Here's the drawing with two shaded views (mm, measured from the low corner). I have some questions. Coordinates: 2 decimals unless noted, no trailing zeros. Write each loop counter-clockwise with the first axis right and the second up, starting at its lowest first coordinate (ties: lowest second). Pieces come first, ordered by that corner, then holes. Notation, with made-up numbers: (64.5, -32) -> (99.5, -32) arc R17 ccw to (99.5, -11) -> close; hole circle Ø5 at (74, -20). An arc over 180 degrees is marked (long way). Use one line per item in the form item = value.
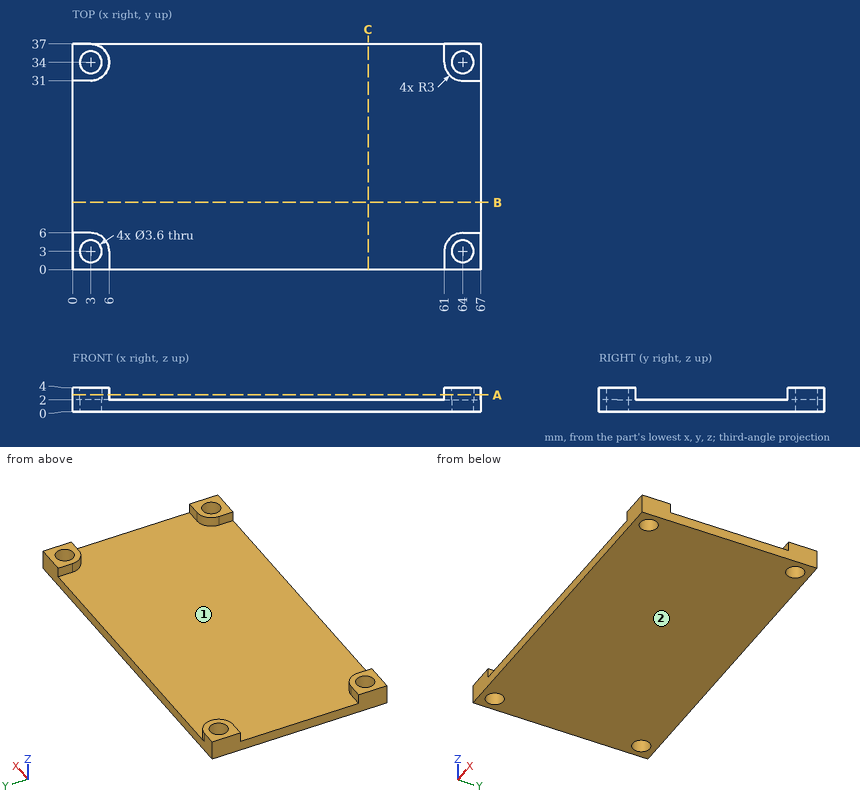
Q1. Suppose I cut it at B-B (y = 11). Write out the boundary of the cut face in (x, z), then the cut area to 3 significant figures.
Return value:
outline = (0, 0) -> (67, 0) -> (67, 2) -> (0, 2) -> close
area = 134 mm2
Q2. Suppose I cut it at C-C (x = 48.5). Write out the boundary of the cut face in (y, z).
Return value:
outline = (0, 0) -> (37, 0) -> (37, 2) -> (0, 2) -> close
Q3. If I drill on line 1 (Y direction, x = 64, z = 3.05); line 2 (Y direction, x = 3, z = 0.95); line 3 (X direction, y = 34, z = 1), over which ranges is the centre line in solid material (lowest first)? Write a range as from..to.
Return value:
line_1 = 0..1.2, 4.8..6, 31..32.2, 35.8..37
line_2 = 0..1.2, 4.8..32.2, 35.8..37
line_3 = 0..1.2, 4.8..62.2, 65.8..67
Q4. Thinking about a two-plate mould opening in X: for the marked faces 1 and 2, which applies, released by +X, released by -X, zero draft, split by the parting line, or undercut?
Return value:
face_1 = undercut
face_2 = zero draft
Q5. Will this pin go through, and if not, where does the flat tip stop? pin 1 (8 mm diameter, centred on x = 55.5, y = 8.5, fed in from +Z).
Return value:
pin_1 = 2
Q6. Suppose I cut it at A-A (z = 2.8). Write out the boundary of the cut face in (x, y).
Return value:
outline = (0, 0) -> (6, 0) -> (6, 3) arc R3 ccw to (3, 6) -> (0, 6) -> close; (0, 31) -> (3, 31) arc R3 ccw to (3, 37) -> (0, 37) -> close; (61, 0) -> (67, 0) -> (67, 6) -> (64, 6) arc R3 ccw to (61, 3) -> close; (61, 34) arc R3 ccw to (64, 31) -> (67, 31) -> (67, 37) -> (61, 37) -> close; hole circle Ø3.6 at (3, 3); hole circle Ø3.6 at (3, 34); hole circle Ø3.6 at (64, 3); hole circle Ø3.6 at (64, 34)
